CAD build for the part. Positions are in the model's coordinates, mm. Face numbers are marked on the shaded views. A direction names the side the tool comes from. Coordinates: 2 decimals unless noted, no trailing zeros. Loops run counter-clockwise (first coordinate to the right, second up) from the corner with the lowest first, then second, coordinate; pieces in that order, holes last. Notation, with made-up numbers: (33, -22.75) - (78, -22.75) arc R23 cw to (78, -8.75) - close; hole circle Ø2 at (64.5, 53.5). An arc over 180 degrees is marked (long way). Put each result on its own line as item: value.
```python
from build123d import *

# Parameters (mm, degrees)
F0_R        = 38.1
F0_W        = 4.1789766401
F0_H        = 8.0406331347
F0_W_2      = 4.8754736781
F0_H_2      = 9.433625348
F0_W_3      = 4.5272270218
F0_H_3      = 9.2595015542
F1_DEPTH    = 7.62
F2_R        = 7.61999
F3_DEPTH    = 10.16
F4_T1_DEPTH = 26.1760218962
F4_T3_DEPTH = 26.1760218962
F4_T5_DEPTH = 26.5242722779
F4_T7_DEPTH = 26.8725189342


# Not quite as in the source:
# - a fillet or chamfer that OpenCascade refuses, or shapes differently, is made with other operations: its cross-section is extruded or revolved along the edge and cut away or added
# - a fillet or chamfer is up to 0.001 mm smaller than in the source, because OpenCascade refuses the exact size


with BuildPart() as f1:
    # F0 (on Top) → F1 (new body)
    with BuildSketch(Plane.XY):
        Circle(F0_R)
        with Locations((-14.8876057938, -18.8208604642)):
            Rectangle(F0_W, F0_H, mode=Mode.SUBTRACT)
        with Locations((14.5393563434, -18.8208604642)):
            Rectangle(F0_W, F0_H, mode=Mode.SUBTRACT)
        with Locations((-15.2358543128, 18.1243643575)):
            Rectangle(F0_W_2, F0_H_2, mode=Mode.SUBTRACT)
        with Locations((14.5393586718, 18.2114262544)):
            Rectangle(F0_W_3, F0_H_3, mode=Mode.SUBTRACT)
    extrude(amount=F1_DEPTH)

    # F2 (radius 7.62 in the source; OpenCascade refuses exactly that, so slightly less here)
    f2_edges = [f1.edges().sort_by_distance(p)[0] for p in [
        (-38.1, 0, 7.62),
    ]]
    fillet(f2_edges, radius=F2_R)

    # F0 (on Top) → F3 (join)
    with BuildSketch(Plane.XY):
        with Locations((-15.2358543128, 18.1243643575)):
            Rectangle(F0_W_2, F0_H_2)
        with Locations((14.5393586718, 18.2114262544)):
            Rectangle(F0_W_3, F0_H_3)
        with Locations((14.5393563434, -18.8208604642)):
            Rectangle(F0_W, F0_H)
        with Locations((-14.8876057938, -18.8208604642)):
            Rectangle(F0_W, F0_H)
    extrude(amount=F3_DEPTH)

    # F4: fillet of radius 5.08 on 8 edges, made by hand

    # F4_s2 → F4_t1 (cut)
    with BuildSketch(Plane.YZ.offset(-27.9756167419)):
        with BuildLine():
            ThreePointArc((-22.8411770315, 7.62), (-20.9817679803, 9.4794090512), (-18.4417679803, 10.16))
            Line((-18.4417679803, 10.16), (-22.8411770315, 10.16))
            Line((-22.8411770315, 10.16), (-22.8411770315, 7.62))
        make_face()
        with BuildLine():
            ThreePointArc((-14.8005438969, 7.62), (-16.6599529481, 9.4794090512), (-19.1999529481, 10.16))
            Line((-19.1999529481, 10.16), (-14.8005438969, 10.16))
            Line((-14.8005438969, 10.16), (-14.8005438969, 7.62))
        make_face()
    extrude(amount=F4_T1_DEPTH, mode=Mode.SUBTRACT)

    # F4_s4 → F4_t3 (cut)
    with BuildSketch(Plane.YZ.offset(1.4513453953)):
        with BuildLine():
            ThreePointArc((-22.8411770315, 7.62), (-20.9817679803, 9.4794090512), (-18.4417679803, 10.16))
            Line((-18.4417679803, 10.16), (-22.8411770315, 10.16))
            Line((-22.8411770315, 10.16), (-22.8411770315, 7.62))
        make_face()
        with BuildLine():
            ThreePointArc((-14.8005438969, 7.62), (-16.6599529481, 9.4794090512), (-19.1999529481, 10.16))
            Line((-19.1999529481, 10.16), (-14.8005438969, 10.16))
            Line((-14.8005438969, 10.16), (-14.8005438969, 7.62))
        make_face()
    extrude(amount=F4_T3_DEPTH, mode=Mode.SUBTRACT)

    # F4_s6 → F4_t5 (cut)
    with BuildSketch(Plane.YZ.offset(1.2772225328)):
        with BuildLine():
            ThreePointArc((13.5816754773, 7.62), (15.4410845286, 9.4794090512), (17.9810845286, 10.16))
            Line((17.9810845286, 10.16), (13.5816754773, 10.16))
            Line((13.5816754773, 10.16), (13.5816754773, 7.62))
        make_face()
        with BuildLine():
            ThreePointArc((22.8411770315, 7.62), (20.9817679803, 9.4794090512), (18.4417679803, 10.16))
            Line((18.4417679803, 10.16), (22.8411770315, 10.16))
            Line((22.8411770315, 10.16), (22.8411770315, 7.62))
        make_face()
    extrude(amount=F4_T5_DEPTH, mode=Mode.SUBTRACT)

    # F4_s8 → F4_t7 (cut)
    with BuildSketch(Plane.YZ.offset(-28.6721137799)):
        with BuildLine():
            ThreePointArc((13.4075516835, 7.62), (15.2669607347, 9.4794090512), (17.8069607347, 10.16))
            Line((17.8069607347, 10.16), (13.4075516835, 10.16))
            Line((13.4075516835, 10.16), (13.4075516835, 7.62))
        make_face()
        with BuildLine():
            ThreePointArc((22.8411770315, 7.62), (20.9817679803, 9.4794090512), (18.4417679803, 10.16))
            Line((18.4417679803, 10.16), (22.8411770315, 10.16))
            Line((22.8411770315, 10.16), (22.8411770315, 7.62))
        make_face()
    extrude(amount=F4_T7_DEPTH, mode=Mode.SUBTRACT)


solid = f1.part
```
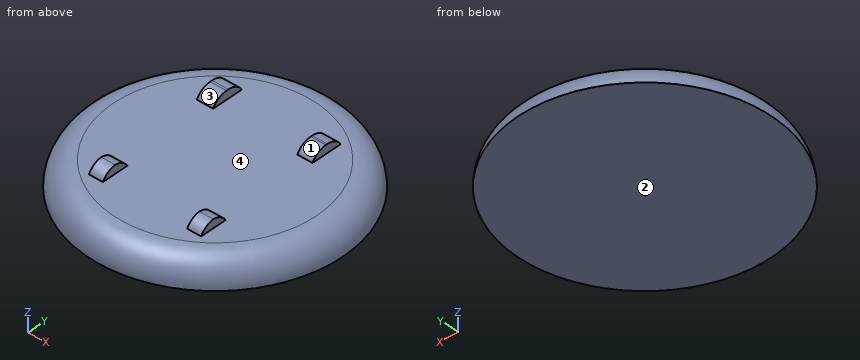
Q1. Mould opens along X. For the marked faces 3 and 4 say: +X half, -X half, draft (parallel to the pull), parting line (faces both ways), or undercut.
Determined:
face 3: draft
face 4: undercut
Q2. Slice it at C-C, the plane z = 2. Give the cut face in (x, y), then the cut area to 3 significant figures.
Determined:
outline: circle Ø75.67 at (0, 0)
area: 4,500 mm2
Q3. Tool access for the marked faces 1 and 2: list every direction of +Z, -Z, +X, -X, +Y, -Y with a clear straight run to the whole face (end or side of a thin tool).
Determined:
face 1: +Z, +X
face 2: -Z, +X, -X, +Y, -Y
Q4. Slice it at A-A, the plane z = 8.75. Give the cut face in (x, y).
Determined:
outline: (-17.67, 14.29) - (-12.8, 14.29) - (-12.8, 21.95) - (-17.67, 21.95) - close; (-16.98, -21.95) - (-12.8, -21.95) - (-12.8, -15.69) - (-16.98, -15.69) - close; (12.28, 14.47) - (16.8, 14.47) - (16.8, 21.95) - (12.28, 21.95) - close; (12.45, -21.95) - (16.63, -21.95) - (16.63, -15.69) - (12.45, -15.69) - close
Q5. Pin check, flat tips, straight feed: pin 1 Ø2 at (y, z) = (-1, 6) entering from +X; pin 2 Ø2 at (y, z) = (19, 9.5) entering from +X; pin 3 Ø5 at (x, z) = (10.5, 3.5) entering from +Y. Stop position of each tip, or through.
Determined:
pin 1: x = 36.22
pin 2: x = 16.8
pin 3: y = 36.88
Q6. Wall check: L1, parallel to X at y = -21, z = 8.5; L2, parallel to Z at x = -1.5, y = 15.5; L3, parallel to X at y = 22, z = 2.75. Give the ranges that are in metal, low to high. Write a range as from..to.
Determined:
L1: -16.98..-12.8, 12.45..16.63
L2: 0..7.62
L3: -30.48..30.48
